```python
from build123d import *

# Parameters (mm, degrees)
SKETCH1_R               = 1.5
BOSS_EXTRUDE1_DEPTH     = 82.55
SKETCH3_R               = 2.775
BOSS_EXTRUDE3_DEPTH     = 3.175
SKETCH4_W               = 0.508
SKETCH4_H               = 6.00854879
SKETCH4_W_2             = 6.00854879
SKETCH4_H_2             = 0.508
CUT_EXTRUDE_THIN1_DEPTH = 2.54
FILLET2_R               = 2


with BuildPart() as part:
    # Sketch1 → Boss-Extrude1 (new body)
    with BuildSketch(Plane.XY):
        Circle(SKETCH1_R)
    extrude(amount=BOSS_EXTRUDE1_DEPTH)

    # Sketch3 → Boss-Extrude3 (add)
    with BuildSketch(Plane.XY.offset(82.55)):
        Circle(SKETCH3_R)
    extrude(amount=-BOSS_EXTRUDE3_DEPTH)

    # Sketch4 → Cut-Extrude-Thin1 (cut)
    with BuildSketch(Plane.XY.offset(82.55)):
        Rectangle(SKETCH4_W, SKETCH4_H)
        Rectangle(SKETCH4_W_2, SKETCH4_H_2)
    extrude(amount=-CUT_EXTRUDE_THIN1_DEPTH, mode=Mode.SUBTRACT)

    # Fillet2
    fillet2_edges = [part.edges().sort_by_distance(p)[0] for p in [
        (-1.962221318, 1.962221318, 82.55),
        (-1.962221318, -1.962221318, 82.55),
        (1.962221318, -1.962221318, 82.55),
        (1.962221318, 1.962221318, 82.55),
    ]]
    fillet(fillet2_edges, radius=FILLET2_R)


solid = part.part
```
The model under review builds one solid part; all positions refer to its coordinate system, in mm. A direction names the side the tool comes from. Give positions to 0.01 mm unless a question says otherwise; leave off trailing zeros. Write each loop counter-clockwise with the first axis right and the second up, starting at its lowest first coordinate (ties: lowest second). Pieces come first, ordered by that corner, then holes. Notation, with made-up numbers: M 81,10.25 L 116,10.25 A36 ccw 116,49.25 Z; hole C 43,73.5 d10. An arc over 180 degrees is marked long. Write item = value, one per line. Start each with the question number.
Q1. We need section A-A (z = 47). State the section outline as (x, y) points, plus the area to 3 significant figures.
Q2. For line 1 (Z direction, x = 0.2, y = -1.4); line 2 (Y direction, x = -0.3, z = 79.5); line 3 (Z direction, x = -0.05, y = -2) (3 decimals), list the stretches that pass through material, from the lowest coordinate up.
Q3. Machinability: for faces 4 (the face through (2.65, 0.83, 79.97)), 5 (the face through (1, -0.254, 81)), 6 (the face through (0, 0, 0)), 7 (the face through (1.2, -1.2, 79.375)), 8 (the face through (-0.254, 1, 81)), which of the approach directions +Z, -Z, +X, -X, +Y, -Y give a long, thin tool a straight path to every point of the face, cutting with its end or side? Answer none if there is none.
Q4. Mouldability with a two-part tool opening along X and no side actions: class faces 1 (the face through (1, 0.254, 81)), 2 (the face through (0.254, 1, 81)), 3 (the face through (-1.5, 0.07, 39.13)) as released by +X, released by -X, zero draft, split by the parting line, or undercut.
Q5. Clearance check with flat-ended pins moving along their axes: pin 1 (1.5 mm diameter, centred on y = -0.5, z = 45.5, fed in from +X); pin 2 (1.3 mm diameter, centred on y = -1, z = 81, fed in from -X); pin 3 (3 mm diameter, centred on x = -2, z = 80.5, fed in from +Y); pin 4 (3 mm diameter, centred on x = -0.5, y = 0, fed in from +Z). State where each tip first meets the part, or that it passes through.
Result set:
q1.outline = C 0,0 d3
q1.area = 7.07 mm2
q2.line_1 = 0 to 80.01
q2.line_2 = -2.76 to 2.76
q2.line_3 = 79.375 to 80.01
q3.face_4 = +Z, -Z
q3.face_5 = +Z, +X, -X
q3.face_6 = -Z, +X, -X, +Y, -Y
q3.face_7 = -Z
q3.face_8 = +Z, +Y, -Y
q4.face_1 = zero draft
q4.face_2 = undercut
q4.face_3 = split by the parting line
q5.pin_1 = 1.5
q5.pin_2 = -2.74
q5.pin_3 = 2.73
q5.pin_4 = 82.55
